from build123d import *

# Parameters (mm, degrees)
F0_W     = 38.1
F0_H     = 31.75
F1_DEPTH = 25.4
F2_W     = 23.7869326904
F2_H     = 14.5215898097
F3_DEPTH = 25.4
F5_DEPTH = 25.4


with BuildPart() as f1:
    # F0 (on Front) → F1 (new body)
    with BuildSketch(Plane.XZ):
        with Locations((19.05, 15.875)):
            Rectangle(F0_W, F0_H)
    extrude(amount=F1_DEPTH)

    # F2 (on face) → F3 (cut)
    with BuildSketch(Plane.XY.offset(31.75)):
        with Locations((26.2065336548, -18.1392050952)):
            Rectangle(F2_W, F2_H)
    extrude(amount=-F3_DEPTH, mode=Mode.SUBTRACT)

    # F4 (on face) → F5 (join)
    with BuildSketch(Plane.YZ.offset(38.1)):
        Polygon((-10.8784101903, 31.75), (-25.4, 6.35), (-10.8784101903, 6.35), align=None)
    extrude(amount=-F5_DEPTH)


solid = f1.part
Model file for the job. Use its own axes, mm. A direction names the side the tool comes from. Coordinates: 2 decimals unless noted, no trailing zeros. Write each loop counter-clockwise with the first axis right and the second up, starting at its lowest first coordinate (ties: lowest second). Pieces come first, ordered by that corner, then holes. Notation, with made-up numbers: (9.5, 73) -> (62.5, 73) arc R15 ccw to (62.5, 101) -> close; hole circle Ø11 at (84.25, 57.25). An arc over 180 degrees is marked (long way). One line per item, written item: value. Start each with the question number.
1) Slice it at B-B on z = 21. Write the cut outline in (x, y), then the cut area to 3 significant figures.
2) Probe probe 1 along X at (y, z) = (-22, 16); probe 2 along Z at (x, y) = (21.5, -14.5); probe 3 along Y at (x, z) = (15, 17.5). List the from-to ranges inside material, lowest first.
3) Flat gauge pins, fed straight in: pin 1 Ø1 at (x, y) = (11.5, -11.5) entering from -Z; pin 2 Ø6 at (x, z) = (31, 28.5) entering from -Y; pin 3 Ø5 at (x, y) = (29.5, -22) entering from +Z. Where does each tip first touch, or does it go through?
4) Slice it at A-A on x = 32.5. Write the cut outline in (y, z).
5) Which spindle directions (+Z, -Z, +X, -X, +Y, -Y) get a long thin tool onto all of the face, cutting with end or side? Do faces 1 (the face through (14.313, -20, 22)), 2 (the face through (10, -25.4, 13)). Say none if no direction does.
6) Slice it at C-C on y = -21.25. Write the cut outline in (x, z).
Answers follow:
1. outline: (0, -25.4) -> (14.31, -25.4) -> (14.31, -17.02) -> (38.1, -17.02) -> (38.1, 0) -> (0, 0) -> close
1. area: 769 mm2
2. probe 1: 0 to 14.31
2. probe 2: 0 to 25.42
2. probe 3: -19.03 to 0
3. pin 1: z = 0
3. pin 2: y = -14.45
3. pin 3: z = 16.67
4. outline: (-25.4, 0) -> (0, 0) -> (0, 31.75) -> (-10.88, 31.75) -> (-25.4, 6.35) -> close
5. face 1: +Z, +X, -Y
5. face 2: +Z, -Z, +X, -X, -Y
6. outline: (0, 0) -> (38.1, 0) -> (38.1, 13.61) -> (14.31, 13.61) -> (14.31, 31.75) -> (0, 31.75) -> close
